```python
from build123d import *

# Parameters (mm, degrees)
F1_DEPTH  = 76.2
F2_R      = 12.7
F3_DEPTH  = 76.201
F5_DEPTH  = 25.401
F7_R      = 19.05
F8_DEPTH  = 6.35
F12_START = -69.85
F12_DEPTH = 12.7
F13_R     = 38.1
F14_SIZE  = 1.524
F16_DEPTH = 6.35
F17_R     = 2.54


# Not quite as in the source:
# - a pattern or mirror of a feature is missing from the dataset's text; its kind, count and spacing are read off the source's solid


with BuildPart() as f1:
    # F0 (on Front) → F1 (new body, symmetric)
    with BuildSketch(Plane.XZ):
        Polygon((0, 0), (-50.8, 0), (-50.8, -25.4), (25.4, -25.4), (25.4, 127), (0, 127), align=None)
    extrude(amount=F1_DEPTH, both=True)

    # F2 (on face) → F3 (cut, through all)
    with BuildSketch(Plane.YZ.offset(25.4)):
        with Locations((0, 88.9)):
            Circle(F2_R)
    extrude(amount=-F3_DEPTH, mode=Mode.SUBTRACT)

    # F4 (on face) → F5 (cut, through all)
    with BuildSketch(Plane.XY):
        with BuildLine():
            Line((-50.8, -12.7), (-38.1, -12.7))
            ThreePointArc((-38.1, -12.7), (-25.4, 0), (-38.1, 12.7))
            Line((-38.1, 12.7), (-50.8, 12.7))
            Line((-50.8, 12.7), (-50.8, -12.7))
        make_face()
    extrude(amount=-F5_DEPTH, mode=Mode.SUBTRACT)

    # F7 (on face) → F8 (cut)
    with BuildSketch(Plane(origin=(0, 0, 0), x_dir=(0, -1, 0), z_dir=(-1, 0, 0))):
        with Locations((0, 88.9)):
            Circle(F7_R)
    f8 = extrude(amount=-F8_DEPTH, mode=Mode.SUBTRACT)

    # F8_copies: F8 across plane
    add(f8.mirror(Plane(origin=(12.7, 0, 0), x_dir=(0, 0, 1), z_dir=(1, 0, 0))), mode=Mode.SUBTRACT)

    # F11 (on offset) → F12 (join)
    with BuildSketch(Plane.XZ.offset(120.65).offset(F12_START)):
        Polygon((0, 0), (0, 76.2), (-25.4, 0), align=None)
    f12 = extrude(amount=-F12_DEPTH)

    # F12_copies: F12 across plane
    add(f12.mirror(Plane.ZX))

    # F13
    f13_edges = [f1.edges().sort_by_distance(p)[0] for p in [
        (12.7, 76.2, 127),
        (12.7, -76.2, 127),
    ]]
    fillet(f13_edges, radius=F13_R)

    # F14
    f14_edges = [f1.edges().sort_by_distance(p)[0] for p in [
        (6.35, -12.7, 88.9),
        (0, 19.05, 88.9),
        (25.4, 19.05, 88.9),
        (19.05, -12.7, 88.9),
    ]]
    chamfer(f14_edges, length=F14_SIZE)

    # F15 (on face) → F16 (join)
    with BuildSketch(Plane.XY):
        with BuildLine():
            Line((-50.8, -19.05), (-38.1, -19.05))
            ThreePointArc((-38.1, -19.05), (-19.05, 0), (-38.1, 19.05))
            Line((-38.1, 19.05), (-50.8, 19.05))
            Line((-50.8, 19.05), (-50.8, 12.7))
            Line((-50.8, 12.7), (-38.1, 12.7))
            ThreePointArc((-38.1, 12.7), (-25.4, 0), (-38.1, -12.7))
            Line((-38.1, -12.7), (-50.8, -12.7))
            Line((-50.8, -12.7), (-50.8, -19.05))
        make_face()
    extrude(amount=F16_DEPTH)

    # F17
    f17_edges = [f1.edges().sort_by_distance(p)[0] for p in [
        (-44.45, 19.05, 0),
        (-12.7, -38.1, 38.1),
        (-12.7, -50.8, 38.1),
        (0, -76.2, 44.45),
        (25.4, -76.2, 31.75),
        (-25.4, -76.2, 0),
        (-12.7, -76.2, -25.4),
        (-25.4, 76.2, 0),
        (-12.7, 76.2, -25.4),
        (25.4, 76.2, 31.75),
        (25.4, 65.040768, 115.840768),
        (25.4, 0, 127),
        (25.4, -65.040768, 115.840768),
        (0, -65.040768, 115.840768),
        (0, 0, 127),
        (0, 65.040768, 115.840768),
        (0, 76.2, 44.45),
        (-12.7, 50.8, 38.1),
        (-12.7, 38.1, 38.1),
        (-44.45, -19.05, 0),
        (-19.05, 0, 0),
    ]]
    fillet(f17_edges, radius=F17_R)


solid = f1.part
```
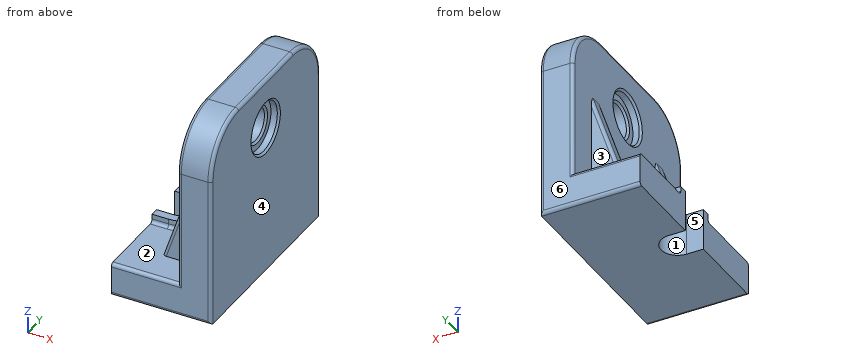
The model under review builds one solid part; all positions refer to its coordinate system, in mm. Face numbers are marked on the shaded views. A direction names the side the tool comes from. Round coordinates to 2 decimals unless told otherwise and drop trailing zeros. Order: outer loops, then holes, each group sorted by start corner. A loop starts at its lowest first (then second) coordinate and runs counter-clockwise, first axis right, second up.
(1) Take a section at B-B, the plane y = -31. State the section outline as (x, z) points, plus the area to 3 significant figures.
Working result:
outline: (-50.8, -25.4) - (25.4, -25.4) - (25.4, 124.46) arc R2.54 ccw to (22.86, 127) - (2.54, 127) arc R2.54 ccw to (0, 124.46) - (0, 0) - (-50.8, 0) - close
area: 5,160 mm2
(2) For P1, Ø4, axis at y = -12, z = 45.5, coming from the -X side; P2, Ø1, axis at x = -15.5, z = 16.5, coming from the -Y side; P3, Ø25, axis at x = -10.5, z = 35.5, coming from the +Y side, all flat-tipped, find the tip position at first contact; note any pin that passes through.
Working result:
P1: stops at x = 0
P2: stops at y = -50.8
P3: stops at y = 76.14
(3) Wall thickness on L1, parallel to Y at x = 21, z = 88; L2, parallel to Z at x = 2.8, y = 0; L3, parallel to Z at x = 12.5, y = 0: over which ranges is each line inside the solid? List them lowest first.
Working result:
L1: y = -76.2 to -19.03, 19.03 to 76.2
L2: z = -25.4 to 69.85, 107.95 to 127
L3: z = -25.4 to 76.2, 101.6 to 127
(4) Tool access review of the marked faces 1, 2 and 3: name each direction out of +Z, -Z, +X, -X, +Y, -Y from which nothing blocks a thin tool from reaching the whole face with its end or side.
Working result:
face 1: +Z, -Z, -X
face 2: +Z
face 3: +Z, -X, +Y
(5) Take a section at C-C, the plane z = -5. State the section outline as (x, y) points, plus the area to 3 significant figures.
Working result:
outline: (-50.8, -76.2) - (22.86, -76.2) arc R2.54 ccw to (25.4, -73.66) - (25.4, 73.66) arc R2.54 ccw to (22.86, 76.2) - (-50.8, 76.2) - (-50.8, 12.7) - (-38.1, 12.7) arc R12.7 cw to (-38.1, -12.7) - (-50.8, -12.7) - close
area: 11,000 mm2
(6) Mouldability with a two-part tool opening along Y and no side actions: class the marked faces 4, 5 and 6 as released by +Y, released by -Y, zero draft, split by the parting line, or undercut.
Working result:
face 4: zero draft
face 5: undercut
face 6: released by +Y
